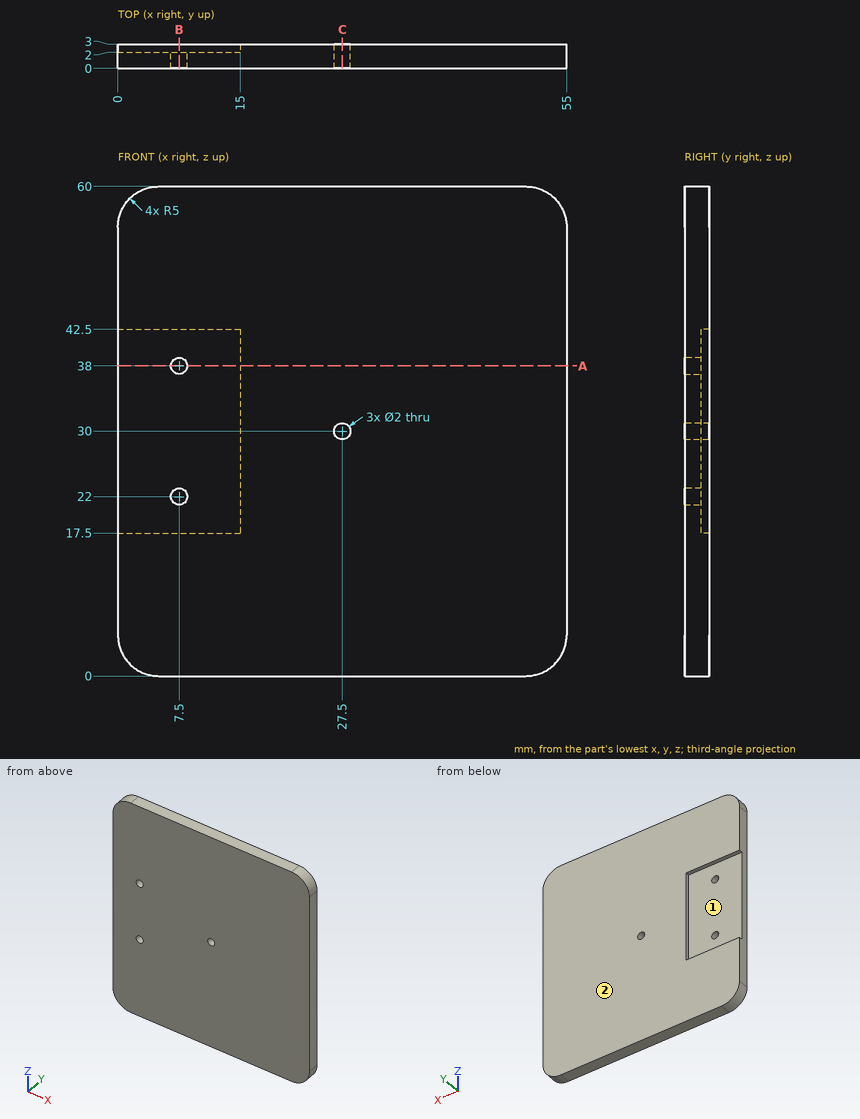
The drawing under review shows one solid part. Ordinate dimensions are in mm from its lowest x, y, z. A direction names the side the tool comes from. Round coordinates to 2 decimals unless told otherwise and drop trailing zeros. Write each loop counter-clockwise with the first axis right and the second up, starting at its lowest first coordinate (ties: lowest second). Pieces come first, ordered by that corner, then holes.
(1) We need section C-C on x = 27.5. Give the boundary of the cut face in (y, z), and give its area (3 significant figures).
(2) We need section B-B on x = 7.5. Give the boundary of the cut face in (y, z).
(3) Machinability: for the marked faces 1 and 2, which of the approach directions +Z, -Z, +X, -X, +Y, -Y give a long, thin tool a straight path to every point of the face, cutting with its end or side? Answer none if there is none.
(4) Insertion check: pin 1 (6 mm diameter, centred on x = 34.5, z = 46, fed in from -Y); pin 2 (0.5 mm diameter, centred on y = 2.5, z = 35.5, fed in from -X); pin 3 (3 mm diameter, centred on x = 7.5, z = 38, fed in from +Y). Each pin has a flat end and moves straight along its axis. Give the tip position at first contact, or say it passes through.
(5) Wall thickness on L1, parallel to X at y = 0.9, z = 38; L2, parallel to Y at x = 6, z = 19; L3, parallel to X at y = 2.25, z = 18.5: over which ranges is each line inside the solid? List them lowest first.
(6) We need section A-A on z = 38. Give the boundary of the cut face in (x, y), and give its area (3 significant figures).
Findings below:
1. outline: (0, 0) - (3, 0) - (3, 29) - (0, 29) - close; (0, 31) - (3, 31) - (3, 60) - (0, 60) - close
1. area: 174 mm2
2. outline: (0, 0) - (3, 0) - (3, 17.5) - (2, 17.5) - (2, 21) - (0, 21) - close; (0, 23) - (2, 23) - (2, 37) - (0, 37) - close; (0, 39) - (2, 39) - (2, 42.5) - (3, 42.5) - (3, 60) - (0, 60) - close
3. face 1: -X, +Y
3. face 2: +Z, -Z, +X, -X, +Y
4. pin 1: stops at y = 0
4. pin 2: stops at x = 15
4. pin 3: stops at y = 2
5. L1: x = 0 to 6.5, 8.5 to 55
5. L2: y = 0 to 2
5. L3: x = 15 to 55
6. outline: (0, 0) - (6.5, 0) - (6.5, 2) - (0, 2) - close; (8.5, 0) - (55, 0) - (55, 3) - (15, 3) - (15, 2) - (8.5, 2) - close
6. area: 146 mm2
